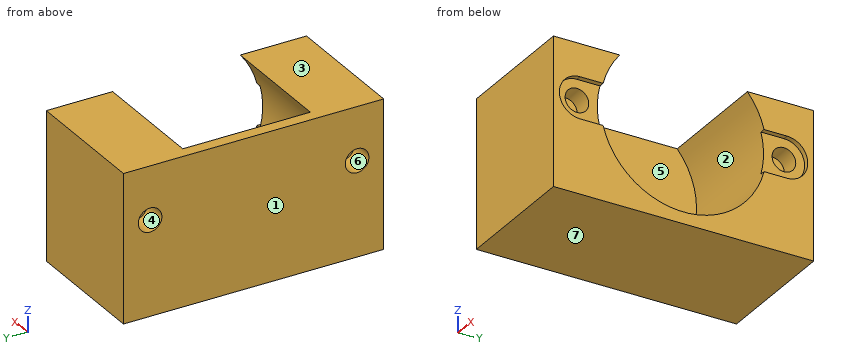
from build123d import *

# Parameters (mm, degrees)
SKETCH_W        = 22
SKETCH_H        = 44
PAD_DEPTH       = 25
SKETCH001_R     = 14.05
POCKET_DEPTH    = 20
SKETCH002_R     = 2
POCKET001_DEPTH = 4.2
POCKET002_DEPTH = 0.9
SKETCH006_R     = 2
POCKET003_DEPTH = 4.2


with BuildPart() as part:
    # Sketch → Pad (new body)
    with BuildSketch(Plane.XY):
        with Locations((-11, 0)):
            Rectangle(SKETCH_W, SKETCH_H)
    extrude(amount=PAD_DEPTH)

    # Sketch001 → Pocket (cut)
    with BuildSketch(Plane.YZ):
        with Locations((0, 16)):
            Circle(SKETCH001_R)
    extrude(amount=-POCKET_DEPTH, mode=Mode.SUBTRACT)

    # Sketch002 → Pocket001 (cut)
    with BuildSketch(Plane.YZ):
        with Locations((-17.5, 16)):
            Circle(SKETCH002_R)
        with Locations((17.5, 16)):
            Circle(SKETCH002_R)
    extrude(amount=-POCKET001_DEPTH, mode=Mode.SUBTRACT)

    # Sketch005 → Pocket002 (cut)
    with BuildSketch(Plane.YZ):
        with BuildLine():
            ThreePointArc((-17.5, 19.5), (-21, 16), (-17.5, 12.5))
            Line((-17.5, 12.5), (17.5, 12.5))
            ThreePointArc((17.5, 12.5), (21, 16), (17.5, 19.5))
            Line((17.5, 19.5), (-17.5, 19.5))
        make_face()
    extrude(amount=-POCKET002_DEPTH, mode=Mode.SUBTRACT)

    # Sketch006 → Pocket003 (cut)
    with BuildSketch(Plane.YZ.offset(-22)):
        with Locations((-17.5, 16)):
            Circle(SKETCH006_R)
        with Locations((17.5, 16)):
            Circle(SKETCH006_R)
    extrude(amount=POCKET003_DEPTH, mode=Mode.SUBTRACT)


solid = part.part
Check sheet for the modelled part. Datum: model origin and axes. Units: mm. Face numbers are marked on the shaded views. A direction names the side the tool comes from. Give positions to 0.01 mm unless a question says otherwise; leave off trailing zeros. Order: outer loops, then holes, each group sorted by start corner. A loop starts at its lowest first (then second) coordinate and runs counter-clockwise, first axis right, second up. Notation, with made-up numbers: (44, 88) - (88, 88) arc R23 ccw to (88, 100) - close; hole circle Ø11 at (24, 46). An arc over 180 degrees is marked (long way). Answer as CSV lines item,"result".
1. Go/stop test with flat-tipped pins: P1, Ø3, axis at y = 17.5, z = 16, coming from the +X side; P2, Ø1.2, axis at y = -17.5, z = 16.5, coming from the -X side; P3, Ø3.5, axis at y = -16.5, z = 17, coming from the +X side. Record where each tip stops, or that it passes through.
Result sheet:
P1,"x = -4.2"
P2,"x = -17.8"
P3,"x = -0.9"
2. Section check A-A (z = 8). Record the boundary of the cut face in (x, y), then the cut area to 3 significant figures.
Result sheet:
outline,"(-22, -22) - (0, -22) - (0, -11.55) - (-20, -11.55) - (-20, 11.55) - (0, 11.55) - (0, 22) - (-22, 22) - close"
area,"506 mm²"
3. Section check B-B (y = 0). Record the boundary of the cut face in (x, z).
Result sheet:
outline,"(-22, 0) - (0, 0) - (0, 1.95) - (-20, 1.95) - (-20, 25) - (-22, 25) - close"
4. Scan lines: probe 1 along Z at (x, y) = (-19.4, 17.5); probe 2 along Y at (x, z) = (-13.5, 16); probe 3 along Y at (x, z) = (-15.5, 11.75). Record each from-to range of solid material in increasing order. Write a range as from..to.
Result sheet:
probe 1,"0..14, 18..25"
probe 2,"-22..-14.05, 14.05..22"
probe 3,"-22..-13.39, 13.39..22"
5. Section check D-D (z = 16). Record the boundary of the cut face in (x, y).
Result sheet:
outline,"(-22, -22) - (0, -22) - (0, -21) - (-0.9, -21) - (-0.9, -19.5) - (-4.2, -19.5) - (-4.2, -15.5) - (-0.9, -15.5) - (-0.9, -14.05) - (-20, -14.05) - (-20, 14.05) - (-0.9, 14.05) - (-0.9, 15.5) - (-4.2, 15.5) - (-4.2, 19.5) - (-0.9, 19.5) - (-0.9, 21) - (0, 21) - (0, 22) - (-22, 22) - (-22, 19.5) - (-17.8, 19.5) - (-17.8, 15.5) - (-22, 15.5) - (-22, -15.5) - (-17.8, -15.5) - (-17.8, -19.5) - (-22, -19.5) - close"
6. Mould release check, pull along Z, two halves, no side actions. Record for the marked faces 1, 2, 3 and 4: released by +Z, released by -Z, zero draft, split by the parting line, or undercut.
Result sheet:
face 1,"zero draft"
face 2,"undercut"
face 3,"released by +Z"
face 4,"undercut"
7. Tool access check on the marked faces 5, 6 and 7. Record the directions out of +Z, -Z, +X, -X, +Y, -Y that give a thin tool (end or side, any length) a straight path to the whole face; none if there is none.
Result sheet:
face 5,"+X"
face 6,"-X"
face 7,"-Z, +X, -X, +Y, -Y"
8. Section check C-C (x = -2.5). Record the boundary of the cut face in (y, z), then the cut area to 3 significant figures.
Result sheet:
outline,"(-22, 0) - (22, 0) - (22, 25) - (10.79, 25) arc R14.05 cw (long way) to (-10.79, 25) - (-22, 25) - close; hole circle Ø4 at (-17.5, 16); hole circle Ø4 at (17.5, 16)"
area,"530 mm²"
